Can you work these out from the drawing? Everything is in mm from the part's minimum corner. A direction names the side the tool comes from. Round coordinates to 2 decimals unless told otherwise and drop trailing zeros. Order: outer loops, then holes, each group sorted by start corner. A loop starts at its lowest first (then second) coordinate and runs counter-clockwise, first axis right, second up. Notation, with made-up numbers: (76.5, 68.5) -> (86.5, 68.5) arc R13 cw to (86.5, 75.5) -> close; hole circle Ø3 at (27.25, 63). An arc over 180 degrees is marked (long way). One line per item, written item: value.
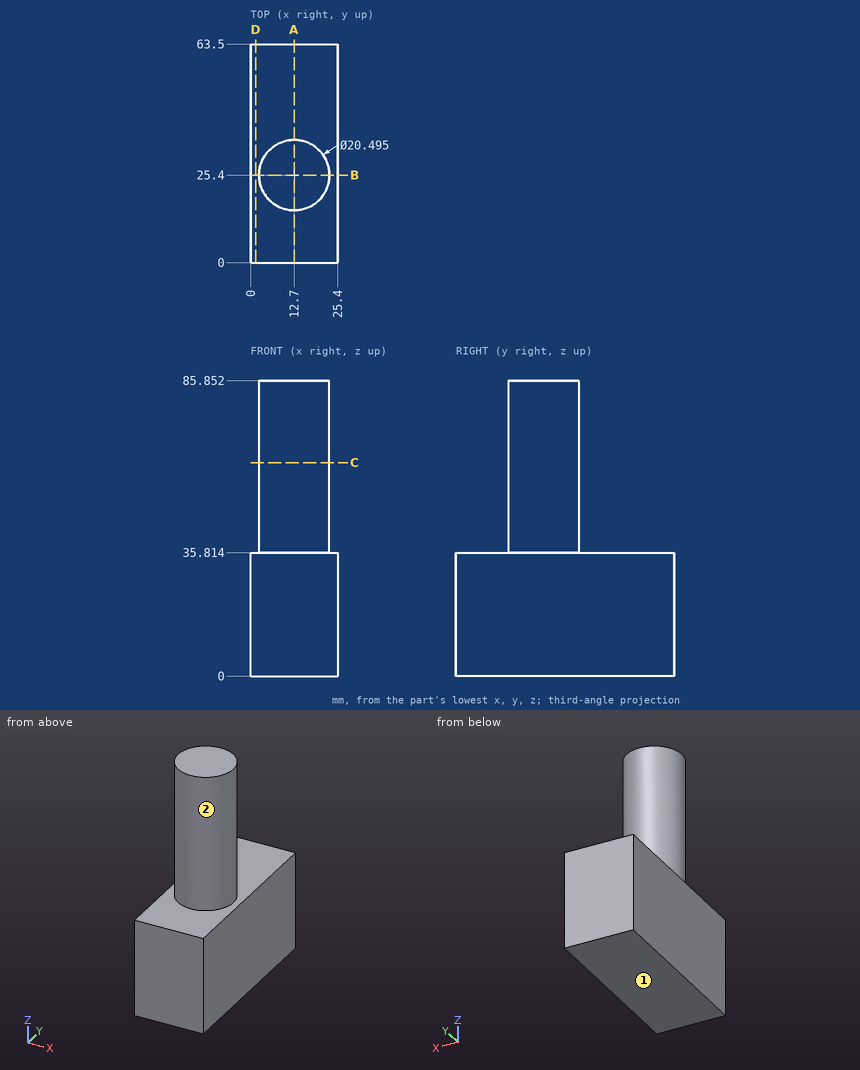
Q1. I want a section at D-D on x = 1.5. List the corners of the cut face in (y, z) for me.
Answers below:
outline: (0, 0) -> (63.5, 0) -> (63.5, 35.81) -> (0, 35.81) -> close
Q2. I want a section at A-A on x = 12.7. List the corners of the cut face in (y, z) for me, plus the area to 3 significant figures.
Answers below:
outline: (0, 0) -> (63.5, 0) -> (63.5, 35.81) -> (35.65, 35.81) -> (35.65, 85.85) -> (15.15, 85.85) -> (15.15, 35.81) -> (0, 35.81) -> close
area: 3,300 mm^2
Q3. On a 3-axis mill with a long thin cutter (end or side, diameter ignored), from which of +Z, -Z, +X, -X, +Y, -Y can I reach the whole of each face in a straight line? I mean the marked faces 1 and 2. Say none if no direction works.
Answers below:
face 1: -Z, +X, -X, +Y, -Y
face 2: +Z
Q4. I want a section at B-B on y = 25.4. List the corners of the cut face in (x, z) for me.
Answers below:
outline: (0, 0) -> (25.4, 0) -> (25.4, 35.81) -> (22.95, 35.81) -> (22.95, 85.85) -> (2.45, 85.85) -> (2.45, 35.81) -> (0, 35.81) -> close
Q5. I want a section at C-C on z = 62. List the corners of the cut face in (x, y) for me (1 decimal), plus the area to 3 significant figures.
Answers below:
outline: circle Ø20.5 at (12.7, 25.4)
area: 330 mm^2
Q6. Will these pins go through, and if not, where does the flat tip stop? pin 1 Ø1 at (x, z) = (8.5, 53.5) entering from +Y; pin 2 Ø5 at (x, z) = (4, 39.5) entering from +Y.
Answers below:
pin 1: y = 34.96
pin 2: y = 33.56
Q7. Please list where these lines run through material, in increasing order: line 1 along Z through (x, y) = (7.5, 53.5); line 2 along Y through (x, z) = (5, 82); line 3 along Y through (x, z) = (13.5, 74).
Answers below:
line 1: 0 to 35.81
line 2: 18.64 to 32.16
line 3: 15.18 to 35.62
